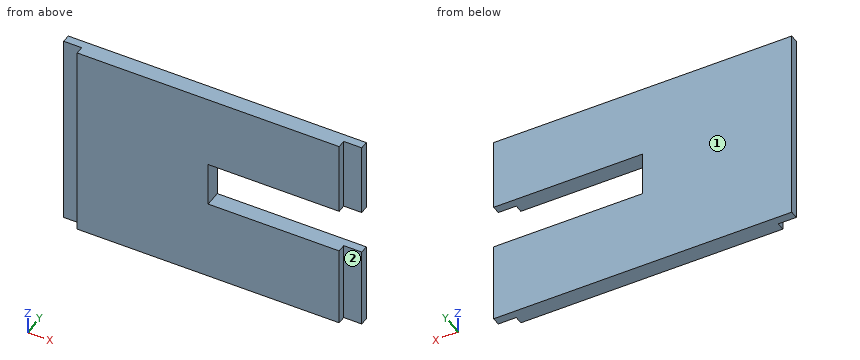
from build123d import *

# Parameters (mm, degrees)
F1_DEPTH = 2.54
F2_W     = 5.588
F2_H     = 22.86
F2_H_2   = 25.4
F2_H_3   = 62.23
F3_DEPTH = 2.54


with BuildPart() as f1:
    # F0 (on Front) → F1 (new body)
    with BuildSketch(Plane.XZ):
        Polygon((40.64, 8.255), (40.64, 31.115), (-40.64, 31.115), (-40.64, -31.115), (40.64, -31.115), (40.64, -5.715), (0, -5.715), (0, 8.255), align=None)
    extrude(amount=F1_DEPTH)

    # F2 (on face) → F3 (join)
    with BuildSketch(Plane(origin=(0, 0, 0), x_dir=(-1, 0, 0), z_dir=(0, 1, 0))):
        with Locations((-43.434, 19.685)):
            Rectangle(F2_W, F2_H)
        Polygon((40.64, 31.115), (-40.64, 31.115), (-40.64, 8.255), (0, 8.255), (0, -5.715), (-40.64, -5.715), (-40.64, -31.115), (40.64, -31.115), align=None)
        with Locations((-43.434, -18.415)):
            Rectangle(F2_W, F2_H_2)
        with Locations((43.434, 0)):
            Rectangle(F2_W, F2_H_3)
    extrude(amount=F3_DEPTH)


solid = f1.part
Work out the finished part from the listing and answer in its coordinate system (mm). Face numbers are marked on the shaded views. A direction names the side the tool comes from. Round coordinates to 2 decimals unless told otherwise and drop trailing zeros. Write each loop counter-clockwise with the first axis right and the second up, starting at its lowest first coordinate (ties: lowest second). Pieces come first, ordered by that corner, then holes. Notation, with made-up numbers: (-1, 32) -> (24, 32) arc R12 ccw to (24, 47) -> close; hole circle Ø2 at (10.25, 36.5). An arc over 180 degrees is marked (long way). Write each question's results on one line, items separated by ' | '.
Item 1: Which of the six approach directions +Z, -Z, +X, -X, +Y, -Y give full straight-line access (tool end or side, diameter ignored) to the marked faces 1 and 2?
Result set:
face 1: +Z, -Z, +X, -X, +Y | face 2: +Z, -Z, +X, -Y
Item 2: A cutting plane is placed at C-C, the plane z = 1. Determine the outline of the cut face in (x, y).
Result set:
outline: (-46.23, 0) -> (-40.64, 0) -> (-40.64, -2.54) -> (0, -2.54) -> (0, 2.54) -> (-46.23, 2.54) -> close
Item 3: Find the intervals of material crossed by line 1 along Z through (x, y) = (14, 0.95) (3 decimals); line 2 along X through (y, z) = (-0.6, -21); line 3 along Y through (x, z) = (-41, 24), in increasing order. Write a range as [from, to].
Result set:
line 1: [-31.115, -5.715], [8.255, 31.115] | line 2: [-40.64, 40.64] | line 3: [0, 2.54]
Item 4: A cutting plane is placed at A-A, the plane x = 32.5. Determine the outline of the cut face in (y, z) (3 decimals), plus the area to 3 significant figures.
Result set:
outline: (-2.54, -31.115) -> (2.54, -31.115) -> (2.54, -5.715) -> (-2.54, -5.715) -> close; (-2.54, 8.255) -> (2.54, 8.255) -> (2.54, 31.115) -> (-2.54, 31.115) -> close | area: 245 mm^2
Item 5: Flat-ended cylindrical pins translate along their axes: P1, Ø3, axis at y = -1, z = 16.5, coming from the +X side; P2, Ø0.8, axis at y = -1, z = -13.5, coming from the -X side; P3, Ø1.5, axis at y = 0, z = 4.5, coming from the +X side; P4, Ø1.7, axis at x = -43, z = -8, coming from the -Y side. Find the tip coordinate at first contact, or state that the pin passes through.
Result set:
P1: x = 46.23 | P2: x = -40.64 | P3: x = 0 | P4: y = 0
Item 6: A cutting plane is placed at B-B, the plane y = 1.65. Determine the outline of the cut face in (x, z) (3 decimals).
Result set:
outline: (-46.228, -31.115) -> (46.228, -31.115) -> (46.228, -5.715) -> (0, -5.715) -> (0, 8.255) -> (46.228, 8.255) -> (46.228, 31.115) -> (-46.228, 31.115) -> close
